Here's how the part is built. I have some questions about the finished solid (model axes, mm). Face numbers are marked on the shaded views. A direction names the side the tool comes from. Coordinates: 2 decimals unless noted, no trailing zeros. Write each loop counter-clockwise with the first axis right and the second up, starting at its lowest first coordinate (ties: lowest second). Pieces come first, ordered by that corner, then holes. Notation, with made-up numbers: M 3.25,12.5 L 42.25,12.5 A17 cw 42.25,27.5 Z; hole C 42,63 d11. An arc over 180 degrees is marked long. Write each question's results on one line, items separated by ' | '. Start each with the question number.
from build123d import *

# Parameters (mm, degrees)
SKETCH1_W             = 260
SKETCH1_H             = 80
BOSS_EXTRUDE1_DEPTH   = 10
EXTRUDE_THIN2_DEPTH   = 80
F_1_0MM_DOWEL_HOLE1_D = 12


with BuildPart() as part:
    # Sketch1 → Boss-Extrude1 (new body)
    with BuildSketch(Plane(origin=(0, 0, 0), x_dir=(1, 0, 0), z_dir=(0, 1, 0))):
        Rectangle(SKETCH1_W, SKETCH1_H)
    extrude(amount=BOSS_EXTRUDE1_DEPTH)

    # Sketch2 → Extrude-Thin2 (add)
    with BuildSketch(Plane.XY.offset(40)):
        Polygon((-30, 30), (-60, 30), (-60, 0), (60, 0), (60, 30), (30, 30), (30, 20), (50, 20), (50, 10), (-50, 10), (-50, 20), (-30, 20), align=None)
    extrude(amount=-EXTRUDE_THIN2_DEPTH)

    # Ø1.0mm Dowel Hole1 (through all)
    with Locations(Plane(origin=(-110, 10, -20), x_dir=(0, 0, 1), z_dir=(0, 1, 0))):
        with Locations((0, 0), (0, 220)):
            Hole(F_1_0MM_DOWEL_HOLE1_D / 2)


solid = part.part
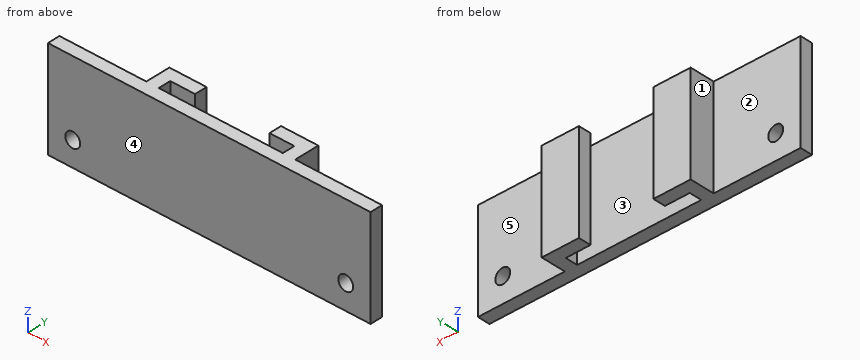
1) I want a section at B-B, the plane x = 110. Write out the boundary of the cut face in (y, z), then the cut area to 3 significant figures.
2) I want a section at C-C, the plane z = -20. Write out the boundary of the cut face in (x, y), then the cut area to 3 significant figures.
3) We'd pull the mould along X, two halves only. Please class the marked faces 1, 2 and 3: pulls with the +X half, pulls with the -X half, needs draft (parallel to the pull), parting line crosses it, or undercut.
4) I want a section at D-D, the plane z = 13.5. Write out the boundary of the cut face in (x, y), then the cut area to 3 significant figures.
5) For pin 1 Ø8 at (y, z) = (24, -3) entering from -X; pin 2 Ø8 at (y, z) = (26.5, -6.5) entering from +X; pin 3 Ø6 at (x, z) = (-67, -5) entering from +Y, each with a flat end and sliding along its axis, tell me the tip position at first contact or that it passes through.
6) Please list where these lines run through material, in increasing order: line 1 (X direction, y = 4.25, z = -20); line 2 (X direction, y = 26.5, z = 14); line 3 (X direction, y = 17.25, z = 36). Write a range as [from, to].
7) For the marked faces 4 and 5, which set-ups out of +Z, -Z, +X, -X, +Y, -Y let a thin tool reach every point of the face, with its end or its side?
8) I want a section at A-A, the plane y = 12.5. Write out the boundary of the cut face in (x, z), then the cut area to 3 significant figures.
Output:
1) outline: M 0,-40 L 10,-40 L 10,-26 L 0,-26 Z; M 0,-14 L 10,-14 L 10,40 L 0,40 Z | area: 680 mm2
2) outline: M -130,0 L -116,0 L -116,10 L -130,10 Z; M -104,0 L 104,0 L 104,10 L 60,10 L 60,30 L 30,30 L 30,20 L 50,20 L 50,10 L -50,10 L -50,20 L -30,20 L -30,30 L -60,30 L -60,10 L -104,10 Z; M 116,0 L 130,0 L 130,10 L 116,10 Z | area: 3,160 mm2
3) face 1: pulls with the -X half | face 2: needs draft | face 3: undercut
4) outline: M -130,0 L 130,0 L 130,10 L 60,10 L 60,30 L 30,30 L 30,20 L 50,20 L 50,10 L -50,10 L -50,20 L -30,20 L -30,30 L -60,30 L -60,10 L -130,10 Z | area: 3,400 mm2
5) pin 1: stops at x = -60 | pin 2: stops at x = 60 | pin 3: stops at y = 10
6) line 1: x = [-130, -116], [-104, 104], [116, 130] | line 2: x = [-60, -30], [30, 60] | line 3: x = [-60, -50], [50, 60]
7) face 4: +Z, -Z, +X, -X, -Y | face 5: +Z, -Z, +X, +Y
8) outline: M -60,-40 L -50,-40 L -50,40 L -60,40 Z; M 50,-40 L 60,-40 L 60,40 L 50,40 Z | area: 1,600 mm2
